Geometry check sheet. Reference: the model listing, model coordinates, mm. Face numbers are marked on the shaded views. A direction names the side the tool comes from. Give positions to 0.01 mm unless a question says otherwise; leave off trailing zeros. Write each loop counter-clockwise with the first axis right and the second up, starting at its lowest first coordinate (ties: lowest second). Pieces come first, ordered by that corner, then holes. Notation, with made-up numbers: (79, 16) - (89, 16) arc R22 ccw to (89, 50) - close; hole circle Ø9 at (60.25, 59). An arc over 180 degrees is marked (long way). One line per question, with ' | ' between items. Start each with the question number.
Q1. Set-up check for the marked faces 5 and 6: record each of +Z, -Z, +X, -X, +Y, -Y from which the full face is reachable in a straight line by a thin tool's end or side.
Q2. Release check for a two-part mould opening along X. For the marked faces 1, 2, 3 and 4 record: +X half, -X half, draft (parallel to the pull), parting line (faces both ways), or undercut.
Q3. Section check A-A on y = -35. Record the boundary of the cut face in (x, z).
Q4. Section check C-C on x = 0. Record the boundary of the cut face in (y, z).
Q5. Gauge pin test, flat ends, axial feed: P1, Ø3, axis at y = -54, z = 1.5, coming from the -X side; P2, Ø4, axis at y = -48.5, z = -1, coming from the -X side; P3, Ø3, axis at x = 9.5, y = -35, coming from the -Z side. Record the tip position at first contact, or that the pin passes through.
Q6. Thickness scan on L1, parallel to X at y = -19.5, z = 5.25; L2, parallel to Z at x = 0, y = -4.65; L3, parallel to Y at x = 2, z = 6.75. Record the ranges inside material, lowest first. Write a range as [from, to].
Q7. Section check B-B on x = -6. Record the boundary of the cut face in (y, z).
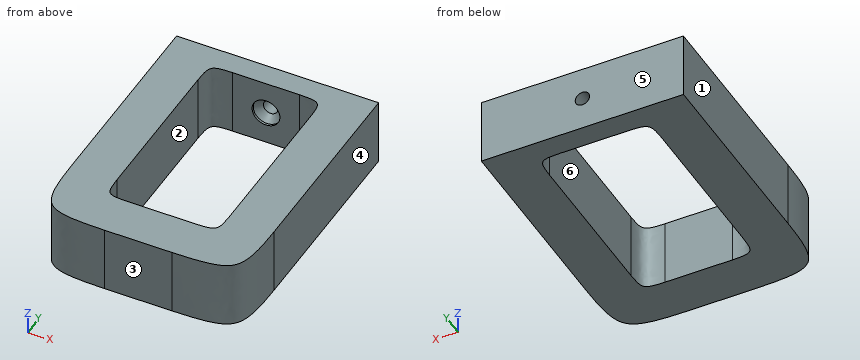
```python
from build123d import *

# Parameters (mm, degrees)
F0_W        = 45
F0_H        = 60
F0_W_2      = 25
F0_H_2      = 45
F1_DEPTH    = 7.5
F4_T1_DEPTH = 15
F5_T1_DEPTH = 90


# Not quite as in the source:
# - a fillet or chamfer that OpenCascade refuses, or shapes differently, is made with other operations: its cross-section is extruded or revolved along the edge and cut away or added


with BuildPart() as f1:
    # F0 (on Top) → F1 (new body, symmetric)
    with BuildSketch(Plane.XY):
        with Locations((0, -30)):
            Rectangle(F0_W, F0_H)
        with Locations((0, -27.5)):
            Rectangle(F0_W_2, F0_H_2, mode=Mode.SUBTRACT)
    extrude(amount=F1_DEPTH, both=True)

    # F2 (on Top) → F3 (revolve, cut)
    with BuildSketch(Plane.XY):
        Polygon((1.6, 0), (0, 0), (0, -5), (3.1, -5), (3.1, -4.5), (1.6, -3), align=None)
    revolve(axis=Axis((0, -2.5, 0), (0, -1, 0)), mode=Mode.SUBTRACT)

    # F4: fillet of radius 5 on 4 edges, made by hand

    # F4_s2 → F4_t1 (join)
    with BuildSketch(Plane.XY.offset(-7.5)):
        with BuildLine():
            add(Edge.make_bspline(
                [(-12.5, -10), (-12.5, -5), (-7.5, -5)],
                knots=[0, 0, 0, 1, 1, 1], degree=2, weights=[1, 2.3333333333, 1]))
            Line((-7.5, -5), (-12.5, -5))
            Line((-12.5, -5), (-12.5, -10))
        make_face()
        with BuildLine():
            add(Edge.make_bspline(
                [(7.5, -5), (12.5, -5), (12.5, -10)],
                knots=[0, 0, 0, 1, 1, 1], degree=2, weights=[1, 2.3333333333, 1]))
            Line((12.5, -10), (12.5, -5))
            Line((12.5, -5), (7.5, -5))
        make_face()
        with BuildLine():
            add(Edge.make_bspline(
                [(-12.5, -45), (-12.5, -50), (-7.5, -50)],
                knots=[0, 0, 0, 1, 1, 1], degree=2, weights=[1, 2.3333333333, 1]))
            Line((-7.5, -50), (-12.5, -50))
            Line((-12.5, -50), (-12.5, -45))
        make_face()
        with BuildLine():
            add(Edge.make_bspline(
                [(12.5, -45), (12.5, -50), (7.5, -50)],
                knots=[0, 0, 0, 1, 1, 1], degree=2, weights=[1, 2.3333333333, 1]))
            Line((7.5, -50), (12.5, -50))
            Line((12.5, -50), (12.5, -45))
        make_face()
    extrude(amount=F4_T1_DEPTH)

    # F5: fillet of radius 15 on 2 edges, made by hand

    # F5_s2 → F5_t1 (cut)
    with BuildSketch(Plane.XY.offset(-45)):
        with BuildLine():
            add(Edge.make_bspline(
                [(-22.5, -45), (-22.5, -60), (-7.5, -60)],
                knots=[0, 0, 0, 1, 1, 1], degree=2, weights=[1, 2.3333333333, 1]))
            Line((-7.5, -60), (-22.5, -60))
            Line((-22.5, -60), (-22.5, -45))
        make_face()
        with BuildLine():
            add(Edge.make_bspline(
                [(22.5, -45), (22.5, -60), (7.5, -60)],
                knots=[0, 0, 0, 1, 1, 1], degree=2, weights=[1, 2.3333333333, 1]))
            Line((7.5, -60), (22.5, -60))
            Line((22.5, -60), (22.5, -45))
        make_face()
    extrude(amount=F5_T1_DEPTH, mode=Mode.SUBTRACT)


solid = f1.part
```
Working result:
1) face 5: +Z, -Z, +X, -X, +Y | face 6: +Z, -Z
2) face 1: -X half | face 2: undercut | face 3: draft | face 4: +X half
3) outline: (-22.5, -7.5) - (-12.5, -7.5) - (-12.5, 7.5) - (-22.5, 7.5) - close; (12.5, -7.5) - (22.5, -7.5) - (22.5, 7.5) - (12.5, 7.5) - close
4) outline: (-60, -7.5) - (-50, -7.5) - (-50, 7.5) - (-60, 7.5) - close; (-5, -7.5) - (0, -7.5) - (0, -1.6) - (-3, -1.6) - (-4.5, -3.1) - (-5, -3.1) - close; (-5, 3.1) - (-4.5, 3.1) - (-3, 1.6) - (0, 1.6) - (0, 7.5) - (-5, 7.5) - close
5) P1: stops at x = -22.18 | P2: stops at x = -22.49 | P3: passes through
6) L1: x = [-22.5, -12.5], [12.5, 22.5] | L2: z = [-7.5, -3.1], [3.1, 7.5] | L3: y = [-60, -50], [-5, 0]
7) outline: (-60, -7.5) - (-50, -7.5) - (-50, 7.5) - (-60, 7.5) - close; (-5, -7.5) - (0, -7.5) - (0, 7.5) - (-5, 7.5) - close
